Geometry check sheet. Reference: the model listing, model coordinates, mm. Face numbers are marked on the shaded views. A direction names the side the tool comes from. Coordinates: 2 decimals unless noted, no trailing zeros. Order: outer loops, then holes, each group sorted by start corner. A loop starts at its lowest first (then second) coordinate and runs counter-clockwise, first axis right, second up.
```python
from build123d import *

# Parameters (mm, degrees)
BOSS_EXTRUDE1_DEPTH = 1
SKETCH3_R           = 3.15
BOSS_EXTRUDE2_DEPTH = 5.4
FILLET1_R           = 0.3
SKETCH4_W           = 0.65
SKETCH4_H           = 2.6
BOSS_EXTRUDE3_DEPTH = 0.3
BOSS_EXTRUDE4_DEPTH = 0.01


with BuildPart() as part:
    # Sketch2 → Boss-Extrude1 (new body)
    with BuildSketch(Plane(origin=(0, 0, 0), x_dir=(1, 0, 0), z_dir=(0, 1, 0))):
        Polygon((3.3, -3.3), (-3.3, -3.3), (-3.3, 2.25), (-2.25, 3.3), (2.25, 3.3), (3.3, 2.25), align=None)
    extrude(amount=BOSS_EXTRUDE1_DEPTH)

    # Sketch3 → Boss-Extrude2 (add)
    with BuildSketch(Plane(origin=(0, 0, 0), x_dir=(1, 0, 0), z_dir=(0, 1, 0))):
        Circle(SKETCH3_R)
    extrude(amount=BOSS_EXTRUDE2_DEPTH)

    # Fillet1
    fillet1_edges = [part.edges().sort_by_distance(p)[0] for p in [
        (-3.15, 5.4, 0),
    ]]
    fillet(fillet1_edges, radius=FILLET1_R)

    # Sketch4 → Boss-Extrude3 (add)
    with BuildSketch(Plane(origin=(0, 0, 0), x_dir=(1, 0, 0), z_dir=(0, 1, 0))):
        with Locations((0, 2.2)):
            Rectangle(SKETCH4_W, SKETCH4_H)
        with Locations((0, -2.2)):
            Rectangle(SKETCH4_W, SKETCH4_H)
    extrude(amount=BOSS_EXTRUDE3_DEPTH)

    # Sketch5 → Boss-Extrude4 (add)
    with BuildSketch(Plane(origin=(0, 5.4, 0), x_dir=(1, 0, 0), z_dir=(0, 1, 0))):
        with BuildLine():
            Line((-2.439908144, -1.472870752), (2.439908144, -1.472870752))
            ThreePointArc((2.439908144, -1.472870752), (0, -2.85), (-2.439908144, -1.472870752))
        make_face()
    extrude(amount=BOSS_EXTRUDE4_DEPTH)


solid = part.part
```
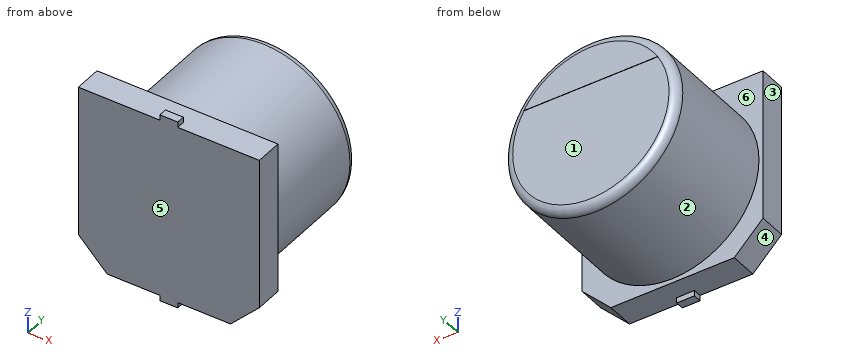
Item 1: Sectioned sample at B-B (z = 0). Record the cut outline in (x, y).
Item 2: Sectioned sample at C-C (y = 3.3). Record the cut outline in (x, z).
Item 3: Thickness scan on line 1 along Y through (x, z) = (3.25, -0.5); line 2 along Y through (x, z) = (-0.5, 0); line 3 along X through (y, z) = (2.85, 1). Record the ranges inside material, lowest first.
Item 4: Depth check by flat-ended pin: P1, Ø1.3, axis at x = 1, z = -1, coming from the +Y side; P2, Ø0.5, axis at x = 1, y = 0.5, coming from the -Z side; P3, Ø1, axis at x = 2.5, z = 2, coming from the -Y side; P4, Ø1.5, axis at x = -1, y = 3, coming from the +Z side. Enter the tip coordinate at first touch or a pass-through.
Item 5: Tool access check on the marked faces 1, 2 and 3. Record the directions out of +Z, -Z, +X, -X, +Y, -Y that give a thin tool (end or side, any length) a straight path to the whole face; none if there is none.
Item 6: Release check for a two-part mould opening along Y. For the marked faces 4, 5 and 6 record: pulls with the +Y half, pulls with the -Y half, needs draft (parallel to the pull), parting line crosses it, or undercut.
Geometry check:
1. outline: (-3.3, 0) - (3.3, 0) - (3.3, 1) - (3.15, 1) - (3.15, 5.1) arc R0.3 ccw to (2.85, 5.4) - (-2.85, 5.4) arc R0.3 ccw to (-3.15, 5.1) - (-3.15, 1) - (-3.3, 1) - close
2. outline: circle Ø6.3 at (0, 0)
3. line 1: y = 0 to 1
3. line 2: y = 0 to 5.4
3. line 3: x = -2.99 to 2.99
4. P1: stops at y = 5.4
4. P2: stops at z = -3.3
4. P3: stops at y = 0
4. P4: stops at z = 3.14
5. face 1: -Z, +X, -X, +Y
5. face 2: +Y
5. face 3: +Z, -Z, -X, +Y, -Y
6. face 4: needs draft
6. face 5: pulls with the -Y half
6. face 6: pulls with the +Y half
